```python
from build123d import *

# Parameters (mm, degrees)
F0_R      = 1.4
F1_DEPTH  = 8
F3_DEPTH  = 54.07728
F5_DEPTH  = 51.401
F6_R      = 2
F8_DEPTH  = 4
F9_R      = 1.4
F10_DEPTH = 4
F11_W     = 2
F11_H     = 6.6
F12_DEPTH = 6


with BuildPart() as f1:
    # F0 (on Top) → F1 (new body)
    with BuildSketch(Plane.XY):
        with BuildLine():
            Line((46.7, 44.37628), (-4.7, 44.37628))
            Line((-4.7, 44.37628), (-4.7, -0.02469))
            ThreePointArc((-4.7, -0.02469), (-1.8661673111, -6.8661673111), (4.97531, -9.7))
            Line((4.97531, -9.7), (37.02469, -9.7))
            ThreePointArc((37.02469, -9.7), (43.8661673111, -6.8661673111), (46.7, -0.02469))
            Line((46.7, -0.02469), (46.7, 44.37628))
        make_face()
        with BuildLine():
            Line((7.7, 38.94554), (7.7, 42.94554))
            Line((7.7, 42.94554), (34.3, 42.94554))
            Line((34.3, 42.94554), (34.3, 38.94554))
            ThreePointArc((34.3, 38.94554), (35.4715728753, 36.1171128753), (38.3, 34.94554))
            Line((38.3, 34.94554), (42.3, 34.94554))
            Line((42.3, 34.94554), (42.3, -0.3))
            Line((42.3, -0.3), (-0.3, -0.3))
            Line((-0.3, -0.3), (-0.3, 34.94554))
            Line((-0.3, 34.94554), (3.7, 34.94554))
            ThreePointArc((3.7, 34.94554), (6.5284271247, 36.1171128753), (7.7, 38.94554))
        make_face(mode=Mode.SUBTRACT)
        with Locations((3.7, 38.94554)):
            Circle(F0_R, mode=Mode.SUBTRACT)
        with Locations((38.3, 38.94554)):
            Circle(F0_R, mode=Mode.SUBTRACT)
    extrude(amount=F1_DEPTH)

    # F2 (on face) → F3 (cut, through all)
    with BuildSketch(Plane(origin=(0, 44.37628, 0), x_dir=(-1, 0, 0), z_dir=(0, 1, 0))):
        Polygon((4.7, 1), (4.7, 8), (2.7, 8), align=None)
        Polygon((-44.7, 8), (-46.7, 8), (-46.7, 1), align=None)
    extrude(amount=-F3_DEPTH, mode=Mode.SUBTRACT)

    # F4 (on face) → F5 (cut, through all)
    with BuildSketch(Plane(origin=(-4.7, 0, 0), x_dir=(0, -1, 0), z_dir=(-1, 0, 0))):
        Polygon((9.7, 8), (1.7, 8), (9.7, 1), align=None)
    extrude(amount=-F5_DEPTH, mode=Mode.SUBTRACT)

    # F6
    f6_edges = [f1.edges().sort_by_distance(p)[0] for p in [
        (7.7, 42.94554, 4),
        (34.3, 42.94554, 4),
        (42.3, 34.94554, 4),
        (-0.3, 34.94554, 4),
    ]]
    fillet(f6_edges, radius=F6_R)

    # F7 (on face) → F8 (cut)
    with BuildSketch(Plane.XY.offset(8)):
        with BuildLine():
            Line((9.7, 42.94554), (3.7, 42.94554))
            ThreePointArc((3.7, 42.94554), (0.8715728753, 41.7739671247), (-0.3, 38.94554))
            Line((-0.3, 38.94554), (-0.3, 32.94554))
            ThreePointArc((-0.3, 32.94554), (0.2857864376, 34.3597535624), (1.7, 34.94554))
            Line((1.7, 34.94554), (3.7, 34.94554))
            ThreePointArc((3.7, 34.94554), (6.5284271247, 36.1171128753), (7.7, 38.94554))
            Line((7.7, 38.94554), (7.7, 40.94554))
            ThreePointArc((7.7, 40.94554), (8.2857864376, 42.3597535624), (9.7, 42.94554))
        make_face()
        with BuildLine():
            Line((38.3, 42.94554), (32.3, 42.94554))
            ThreePointArc((32.3, 42.94554), (33.7142135624, 42.3597535624), (34.3, 40.94554))
            Line((34.3, 40.94554), (34.3, 38.94554))
            ThreePointArc((34.3, 38.94554), (35.4715728753, 36.1171128753), (38.3, 34.94554))
            Line((38.3, 34.94554), (40.3, 34.94554))
            ThreePointArc((40.3, 34.94554), (41.7142135624, 34.3597535624), (42.3, 32.94554))
            Line((42.3, 32.94554), (42.3, 38.94554))
            ThreePointArc((42.3, 38.94554), (41.1284271247, 41.7739671247), (38.3, 42.94554))
        make_face()
        with BuildLine():
            Line((7.7, -0.3), (-0.3, -0.3))
            Line((-0.3, -0.3), (-0.3, -4.3))
            ThreePointArc((-0.3, -4.3), (0.8715728753, -7.1284271247), (3.7, -8.3))
            Line((3.7, -8.3), (7.7, -8.3))
            Line((7.7, -8.3), (7.7, -0.3))
        make_face()
        with BuildLine():
            Line((42.3, -4.3), (42.3, -0.3))
            Line((42.3, -0.3), (34.3, -0.3))
            Line((34.3, -0.3), (34.3, -8.3))
            Line((34.3, -8.3), (38.3, -8.3))
            ThreePointArc((38.3, -8.3), (41.1284271247, -7.1284271247), (42.3, -4.3))
        make_face()
    extrude(amount=-F8_DEPTH, mode=Mode.SUBTRACT)

    # F9 (on face) → F10 (cut, through all)
    with BuildSketch(Plane.XY.offset(4)):
        with Locations((3.7, -3.3)):
            Circle(F9_R)
        with Locations((38.3, -3.3)):
            Circle(F9_R)
    extrude(amount=-F10_DEPTH, mode=Mode.SUBTRACT)

    # F11 (on face) → F12 (cut)
    with BuildSketch(Plane.XY.offset(8)):
        with Locations((11, -5)):
            Rectangle(F11_W, F11_H)
        with Locations((15, -5)):
            Rectangle(F11_W, F11_H)
        with Locations((19, -5)):
            Rectangle(F11_W, F11_H)
        with Locations((31, -5)):
            Rectangle(F11_W, F11_H)
        with Locations((27, -5)):
            Rectangle(F11_W, F11_H)
        with Locations((23, -5)):
            Rectangle(F11_W, F11_H)
    extrude(amount=-F12_DEPTH, mode=Mode.SUBTRACT)


solid = f1.part
```
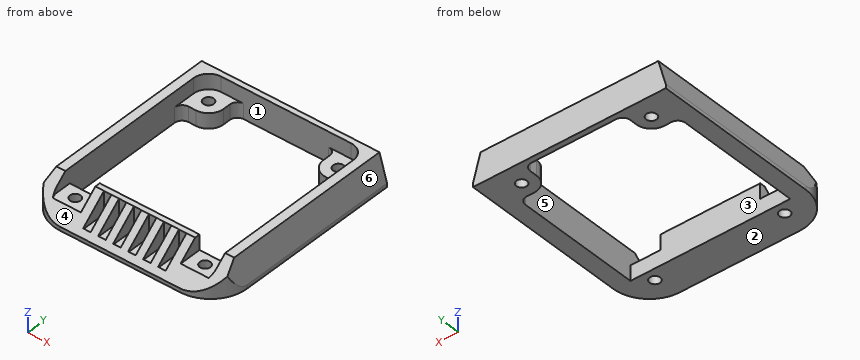
Geometry check sheet. Reference: the model listing, model coordinates, mm. Face numbers are marked on the shaded views. A direction names the side the tool comes from. Coordinates: 2 decimals unless noted, no trailing zeros. Write each loop counter-clockwise with the first axis right and the second up, starting at its lowest first coordinate (ties: lowest second). Pieces come first, ordered by that corner, then holes. Notation, with made-up numbers: M 27,76 L 58,76 A19 cw 58,107 Z; hole C -27,31 d4. An arc over 180 degrees is marked long. One line per item, written item: value. Start each with the question number.
(1) Sectioned sample at A-A, the plane y = 9. Enter the section's corners in (x, z).
(2) Release check for a two-part mould opening along X. For the marked faces 4, 5 and 6 record: released by +X, released by -X, zero draft, split by the parting line, or undercut.
(3) Sectioned sample at C-C, the plane y = -3.3. State how many separate pieces and enclosed holes the cut face has, and give its area (3 significant figures).
(4) Scan lines: line 1 along Y through (x, z) = (38.3, 1.7); line 2 along Y through (x, z) = (3.7, 1.45); line 3 along X through (y, z) = (10, 0.5). Record each from-to range of solid material in increasing order. Write a range as [from, to].
(5) Tool access check on the marked faces 1, 2 and 3. Record the directions out of +Z, -Z, +X, -X, +Y, -Y that give a thin tool (end or side, any length) a straight path to the whole face; none if there is none.
(6) Sectioned sample at B-B, the plane x = 11. Enter the section's corners in (y, z) (3 decimals).
(7) Depth check by flat-ended pin: pin 1 (1 mm diameter, centred on y = -2, z = 7, fed in from +X); pin 2 (0.6 mm diameter, centred on x = 23.5, y = -4, fed in from +Z); pin 3 (5 mm diameter, centred on x = 4.5, y = 35, fed in from +Z). Enter the tip coordinate at first touch or a pass-through.
Filled sheet:
1. outline: M -4.7,0 L -0.3,0 L -0.3,8 L -2.7,8 L -4.7,1 Z; M 42.3,0 L 46.7,0 L 46.7,1 L 44.7,8 L 42.3,8 Z
2. face 4: zero draft
2. face 5: undercut
2. face 6: released by +X
3. separate pieces: 3
3. enclosed holes: 0
3. area: 209 mm²
4. line 1: [-8.9, -4.7], [-1.9, -0.3], [34.95, 37.55], [40.35, 44.38]
4. line 2: [-9.19, -4.7], [-1.9, -0.3], [34.95, 37.55], [40.35, 44.38]
4. line 3: [-4.7, -0.3], [42.3, 46.7]
5. face 1: +Z
5. face 2: -Z, +X, -X, +Y, -Y
5. face 3: +Z, -Z
6. outline: M -9.7,0 L -0.3,0 L -0.3,8 L -1.7,8 L -1.7,2 L -8.3,2 L -8.3,2.225 L -9.7,1 Z; M 42.946,0 L 44.376,0 L 44.376,8 L 42.946,8 Z
7. pin 1: x = 45.13
7. pin 2: z = 2
7. pin 3: z = 4
